Source: CAD feature listing. Evaluate the final solid. Frame: model axes, mm. Face numbers are marked on the shaded views. Round coordinates to 2 decimals unless told otherwise and drop trailing zeros. Order: outer loops, then holes, each group sorted by start corner. A loop starts at its lowest first (then second) coordinate and runs counter-clockwise, first axis right, second up. Notation, with made-up numbers: (-18.5, 85.25) -> (17.5, 85.25) arc R27 ccw to (17.5, 101.25) -> close; hole circle Ø6 at (-17, 37). An arc over 180 degrees is marked (long way). Write item = value, one per line. Start each with the question number.
(1) Draft query along Z for the marked faces 1, 2 and 3. Return one class per face: released by +Z, released by -Z, zero draft, split by the parting line, or undercut.
(2) Cut plane C-C on z = -1.5. Return the cut outline in (x, y).
(3) Contact query for flat-ended pins moving along their axis: pin 1 Ø1 at (y, z) = (-9, -3) entering from -X; pin 2 Ø5 at (x, y) = (-1, -5) entering from -Z; pin 3 Ø1 at (x, z) = (-1, -2) entering from -Y. Output: stop coordinate, or through.
(4) Cut plane A-A on x = 0. Return the cut outline in (y, z), then the cut area to 3 significant figures.
(5) Cut plane B-B on y = -7. Return the cut outline in (x, z).
(6) Ray query, line 1 (Z direction, x = 0, y = -7); line 2 (Z direction, x = 0, y = -13.5); line 3 (Z direction, x = 0.75, y = -7). Return the intervals inside material, ascending.
(7) Cut plane D-D on y = -14.5. Return the cut outline in (x, z).
from build123d import *

# Parameters (mm, degrees)
F0_R     = 3.5
F1_DEPTH = 20
F2_T     = 1
F3_R     = 3.3401010272
F4_DEPTH = 10
F5_R     = 4.5
F6_DEPTH = 10
F7_R     = 2.1745755041
F8_DEPTH = 15
F8_TAPER = -3


with BuildPart() as f1:
    # F0 (on Front) → F1 (new body)
    with BuildSketch(Plane.XZ):
        Circle(F0_R)
    extrude(amount=F1_DEPTH)

    # F2
    f2_openings = [f1.faces().sort_by_distance(p)[0] for p in [
        (0, -20, 0),
    ]]
    offset(amount=F2_T, openings=f2_openings, kind=Kind.INTERSECTION)

    # F3 (on Front) → F4 (join)
    with BuildSketch(Plane.XZ):
        Circle(F3_R)
    extrude(amount=F4_DEPTH)

    # F5 (on Front) → F6 (join)
    with BuildSketch(Plane.XZ):
        Circle(F5_R)
    extrude(amount=-F6_DEPTH)

    # F7 (on Top) → F8 (cut, symmetric)
    with BuildSketch(Plane.XY):
        with Locations((0, 5.7148435153)):
            Circle(F7_R)
    extrude(amount=F8_DEPTH, both=True, taper=F8_TAPER, mode=Mode.SUBTRACT)


solid = f1.part
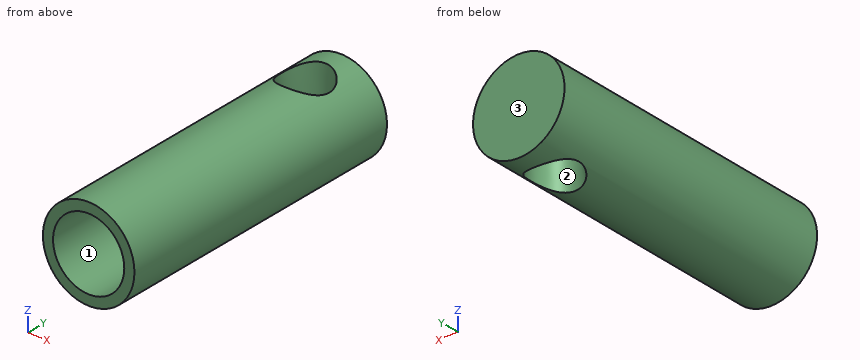
Evaluation:
q1.face_1 = undercut
q1.face_2 = released by -Z
q1.face_3 = zero draft
q2.outline = (-4.24, -20) -> (-3.16, -20) -> (-3.16, 0) -> (-2.98, 0) -> (-2.98, -10) -> (2.98, -10) -> (2.98, 0) -> (3.16, 0) -> (3.16, -20) -> (4.24, -20) -> (4.24, 10) -> (-4.24, 10) -> close; hole circle Ø4.51 at (0, 5.71)
q3.pin_1 = -3.74
q3.pin_2 = -4.5
q3.pin_3 = -10
q4.outline = (-20, -4.5) -> (3.3, -4.5) -> (3.54, 0) -> (3.3, 4.5) -> (-20, 4.5) -> (-20, 3.5) -> (0, 3.5) -> (0, 3.34) -> (-10, 3.34) -> (-10, -3.34) -> (0, -3.34) -> (0, -3.5) -> (-20, -3.5) -> close; (7.89, 0) -> (8.13, -4.5) -> (10, -4.5) -> (10, 4.5) -> (8.13, 4.5) -> close
q4.area = 156 mm^2
q5.outline = circle Ø9 at (0, 0); circle Ø6.68 at (0, 0); hole circle Ø7 at (0, 0)
q6.line_1 = -4.5 to -3.5, -3.34 to 3.34, 3.5 to 4.5
q6.line_2 = -4.5 to -3.5, 3.5 to 4.5
q6.line_3 = -4.44 to -3.42, -3.25 to 3.25, 3.42 to 4.44
q7.outline = circle Ø9 at (0, 0); hole circle Ø7 at (0, 0)
